from build123d import *

# Parameters (mm, degrees)
SKETCH1_R           = 76.2
BOSS_EXTRUDE1_DEPTH = 254
SCALE1_SCALE        = 0.0393701


with BuildPart() as part:
    # Sketch1 → Boss-Extrude1 (new body)
    with BuildSketch(Plane(origin=(0, 0, 0), x_dir=(1, 0, 0), z_dir=(0, 1, 0))):
        with Locations(Location((0, 0, 0), (0, 0, 270))):
            Circle(SKETCH1_R)
    extrude(amount=BOSS_EXTRUDE1_DEPTH)

    # Sketch2 → Revolve3 (revolve)
    with BuildSketch(Plane(origin=(0, 0, 0), x_dir=(0, 0, -1), z_dir=(1, 0, 0)), mode=Mode.PRIVATE) as revolve3_sk:
        with BuildLine():
            Line((0, 371.361992924), (0, 254))
            Line((0, 254), (76.2, 254))
            Line((76.2, 254), (152.4, 254))
            ThreePointArc((152.4, 254), (96.176397031, 338.621276033), (0, 371.361992924))
        make_face()
    revolve(revolve3_sk.sketch.rotate(Axis((0, 254, 0), (0, 1, 0)), 180), axis=Axis((0, 254, 0), (0, 1, 0)))


with BuildPart() as part_1:
    # Scale1: scaled about (0, 215.966552743, 0)
    add(part.part.scale(SCALE1_SCALE).moved(Location((0, 207.463927965, 0))))


solid = part_1.part
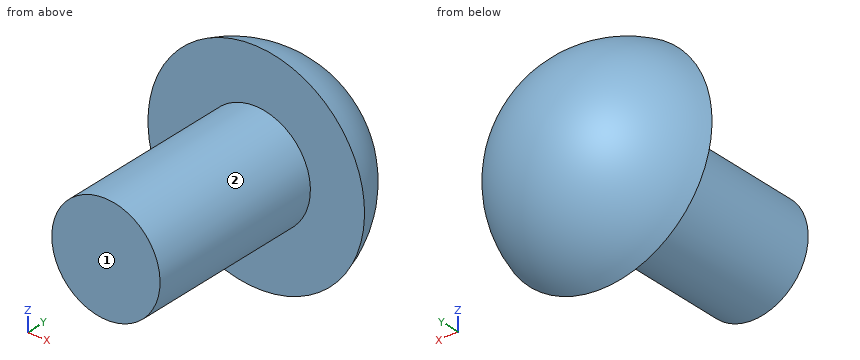
The listing builds one solid part. Answer for the finished solid, in the listing's coordinates (mm). Face numbers are marked on the shaded views. A direction names the side the tool comes from. Give positions to 0.01 mm unless a question says otherwise; leave off trailing zeros. Order: outer loops, then holes, each group sorted by start corner. A loop starts at its lowest first (then second) coordinate and runs counter-clockwise, first axis right, second up. Notation, with made-up numbers: (-17, 7.25) - (-9, 7.25) arc R21 ccw to (-9, 26.25) - close; hole circle Ø11 at (0.5, 18.25). An arc over 180 degrees is marked (long way). One line per item, written item: value. Start each with the question number.
1) Find the intervals of material crossed by L1, parallel to X at y = 213.25, z = -1.25; L2, parallel to Z at x = -2, y = 216; L3, parallel to Y at x = 1, z = 1.25, in increasing order.
2) A cutting plane is placed at A-A on x = 0. Give the vertices of the cut face in (y, z), then the cut area to 3 significant figures.
3) A cutting plane is placed at D-D on z = 4. Give the vertices of the cut face in (x, y), then the cut area to 3 significant figures.
4) Given pin 1 Ø2 at (x, z) = (-2, -4.5) entering from +Y; pin 2 Ø2 at (x, y) = (-4.5, 215.5) entering from -Z; pin 3 Ø3 at (x, y) = (1.5, 219) entering from +Z; pin 4 Ø1.5 at (x, y) = (1.5, 212.5) entering from +Z, each flat-ended and moving along its own axis, determine where each tip first touches the part or whether it passes through.
5) A cutting plane is placed at B-B on y = 216. Give the vertices of the cut face in (x, z).
6) A tool of negligible diameter and unlimited length cuts with its end or side. For the marked faces 1 and 2, from which of +Z, -Z, +X, -X, +Y, -Y can it reach the whole face along a straight path? Write none if from no direction.
7) A cutting plane is placed at C-C on z = 0. Give the vertices of the cut face in (x, y).
Answer sheet:
1. L1: x = -2.73 to 2.73
1. L2: z = -2.24 to 2.24
1. L3: y = 207.46 to 221.87
2. outline: (207.46, -3) - (217.46, -3) - (217.46, -6) arc R6.21 ccw to (217.46, 6) - (217.46, 3) - (207.46, 3) - close
2. area: 101 mm2
3. outline: (-4.47, 217.46) - (4.47, 217.46) arc R4.74 ccw to start
3. area: 20.6 mm2
4. pin 1: stops at y = 220.69
4. pin 2: passes through
4. pin 3: stops at z = 5.89
4. pin 4: stops at z = 2.9
5. outline: circle Ø6 at (0, 0)
6. face 1: +Z, -Z, +X, -X, -Y
6. face 2: -Y
7. outline: (-6, 217.46) - (-3, 217.46) - (-3, 207.46) - (3, 207.46) - (3, 217.46) - (6, 217.46) arc R6.21 ccw to start
